```python
from build123d import *

# Parameters (mm, degrees)
F0_W     = 105
F0_H     = 25
F1_DEPTH = 15
F2_R     = 2.525
F3_DEPTH = 25
F4_W     = 105
F4_H     = 5
F5_DEPTH = 25


with BuildPart() as f1:
    # F0 (on Top) → F1 (new body)
    with BuildSketch(Plane.XY):
        Polygon((-61.220747, -19.834538), (-61.220747, -14.834538), (-96.220747, -14.834538), (-96.220747, -49.834538), (-91.220747, -49.834538), (-91.220747, -19.834538), align=None)
        Polygon((53.779253, -14.834538), (-61.220747, -14.834538), (-61.220747, -19.834538), (-61.220747, -49.834538), (53.779253, -49.834538), align=None)
        with Locations((-3.720747, -32.334538)):
            Rectangle(F0_W, F0_H, mode=Mode.SUBTRACT)
    extrude(amount=F1_DEPTH)

    # F2 (on face) → F3 (cut)
    with BuildSketch(Plane(origin=(-96.220747, 0, 0), x_dir=(0, -1, 0), z_dir=(-1, 0, 0))):
        with Locations((32.334538, 7.5)):
            Circle(F2_R)
    extrude(amount=-F3_DEPTH, mode=Mode.SUBTRACT)

    # F4 (on face) → F5 (cut)
    with BuildSketch(Plane.XZ.offset(19.834538)):
        with Locations((-3.720747, 12.5)):
            Rectangle(F4_W, F4_H)
        with Locations((-3.720747, 7.5)):
            Rectangle(F4_W, F4_H)
    extrude(amount=-F5_DEPTH, mode=Mode.SUBTRACT)


solid = f1.part
```
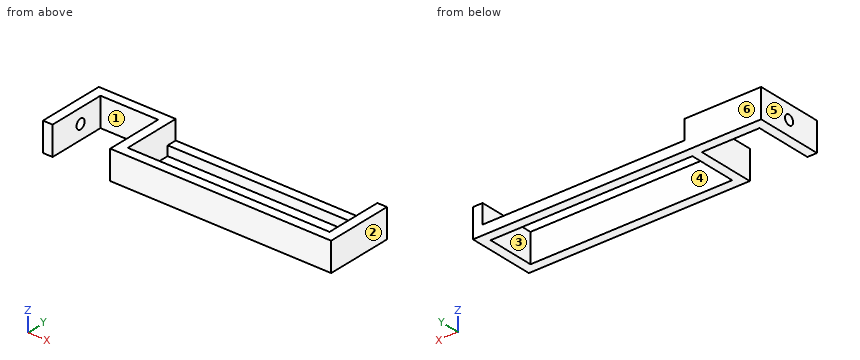
Verification items for the finished model (mm, model axes). Face numbers are marked on the shaded views. A direction names the side the tool comes from. Coordinates: 2 decimals unless noted, no trailing zeros. Order: outer loops, then holes, each group sorted by start corner. A loop starts at its lowest first (then second) coordinate and runs counter-clockwise, first axis right, second up. Notation, with made-up numbers: (17, -31.75) -> (62, -31.75) arc R17 cw to (62, -18.75) -> close; hole circle Ø6 at (74.25, -38.5). An arc over 180 degrees is marked (long way). Put each result on its own line as item: value. Start each with the question number.
1) Cross-section at A-A (x = -13.5). Enter the section's corners in (y, z), plus the area to 4 significant figures.
2) Release check for a two-part mould opening along Y. For the marked faces 3, 4, 5 and 6 record: pulls with the +Y half, pulls with the -Y half, needs draft (parallel to the pull), parting line crosses it, or undercut.
3) Go/stop test with a flat-tipped pin: pin 1 (5.5 mm diameter, centred on x = -7, y = -17, fed in from +Z). Record where the tip stops, or that it passes through.
4) Cross-section at C-C (z = 7.5). Enter the section's corners in (x, y).
5) Cross-section at D-D (x = -75.5). Enter the section's corners in (y, z), plus the area to 3 significant figures.
6) Material ranges on L1, parallel to X at y = -20, z = 14; L2, parallel to X at y = -19, z = 9.5; L3, parallel to Y at x = 46, z = 3.75, recorded low to high.
7) Cross-section at B-B (y = -23.5). Enter the section's corners in (x, z), plus the area to 3 significant figures.
8) Tool access check on the marked faces 1 and 2. Record the directions out of +Z, -Z, +X, -X, +Y, -Y that give a thin tool (end or side, any length) a straight path to the whole face; none if there is none.
Geometry check:
1. outline: (-49.83, 0) -> (-44.83, 0) -> (-44.83, 15) -> (-49.83, 15) -> close; (-19.83, 0) -> (-14.83, 0) -> (-14.83, 5) -> (-19.83, 5) -> close
1. area: 100.0 mm^2
2. face 3: undercut
2. face 4: undercut
2. face 5: needs draft
2. face 6: pulls with the +Y half
3. pin 1: stops at z = 5
4. outline: (-96.22, -49.83) -> (-91.22, -49.83) -> (-91.22, -34.86) -> (-96.22, -34.86) -> close; (-96.22, -29.81) -> (-91.22, -29.81) -> (-91.22, -19.83) -> (-61.22, -19.83) -> (-61.22, -49.83) -> (53.78, -49.83) -> (53.78, -14.83) -> (48.78, -14.83) -> (48.78, -44.83) -> (-56.22, -44.83) -> (-56.22, -14.83) -> (-96.22, -14.83) -> close
5. outline: (-19.83, 0) -> (-14.83, 0) -> (-14.83, 15) -> (-19.83, 15) -> close
5. area: 75.0 mm^2
6. L1: x = -96.22 to -91.22, -61.22 to -56.22, 48.78 to 53.78
6. L2: x = -96.22 to -56.22, 48.78 to 53.78
6. L3: y = -49.83 to -44.83, -19.83 to -14.83
7. outline: (-96.22, 0) -> (-91.22, 0) -> (-91.22, 15) -> (-96.22, 15) -> close; (-61.22, 0) -> (-56.22, 0) -> (-56.22, 15) -> (-61.22, 15) -> close; (48.78, 0) -> (53.78, 0) -> (53.78, 15) -> (48.78, 15) -> close
7. area: 225 mm^2
8. face 1: +Z, -Z, -Y
8. face 2: +Z, -Z, +X, +Y, -Y
